Input: part model. Units: mm. Frame: model coordinates. A direction names the side the tool comes from. Round coordinates to 2 decimals unless told otherwise and drop trailing zeros. Order: outer loops, then holes, each group sorted by start corner. A loop starts at its lowest first (then second) coordinate and runs counter-clockwise, first axis right, second up. Notation, with made-up numbers: (50.5, 25) -> (64.5, 25) arc R7 ccw to (64.5, 38) -> close; hole circle Ø8 at (16.25, 64). An arc over 180 degrees is marked (long way). Use a Markdown table: item, result.
from build123d import *

# Parameters (mm, degrees)
SKETCH2_R                   = 7.9375
SKETCH2_R_2                 = 3.7465
BOSS_EXTRUDE1_DEPTH         = 204.47
FILLET1_R                   = 3.81
CIRPATTERN1_COUNT           = 4
FILLET1_OF_CIRPATTERN1_R    = 3.81
SKETCH3_R                   = 8.636
CUT_EXTRUDE1_DEPTH          = 12.7
CIRPATTERN2_COUNT           = 4
FILLET2_R                   = 2.54
MIRROR1_COPY_1_SKETCH_R     = 8.636
MIRROR1_COPY_1_DEPTH        = 12.7
MIRROR1_COPY_2_SKETCH_R     = 8.636
MIRROR1_COPY_2_DEPTH        = 12.7
MIRROR1_COPY_3_SKETCH_R     = 8.636
MIRROR1_COPY_3_DEPTH        = 12.7
FILLET3_R                   = 2.54
CHAMFER1_SIZE               = 1.27
CHAMFER1_SIZE_2             = 7.202527911
F_3_8_CLEARANCE_HOLE1_D     = 10.0838
F_3_8_CLEARANCE_HOLE1_DEPTH = 54.864
F_3_8_CLEARANCE_HOLE1_TIP   = 3.029479155
CIRPATTERN3_COUNT           = 3
CIRPATTERN3_ANGLE           = 180
CUT_EXTRUDE2_START          = -204.47
SKETCH9_R                   = 52.832
CUT_EXTRUDE2_DEPTH          = 101.788087
SKETCH10_W                  = 4.445
SKETCH10_H                  = 6.796913


with BuildPart() as part:
    # Sketch1 → Revolve1 (revolve)
    with BuildSketch(Plane.XY, mode=Mode.PRIVATE) as revolve1_sk:
        Polygon((44.45, 0), (44.45, 204.47), (50.7238, 204.47), (50.7238, 108.585), (52.832, 108.585), (52.832, 95.885), (50.7238, 95.885), (50.7238, 0), align=None)
    revolve(revolve1_sk.sketch.rotate(Axis((0, 138.931800571, 0), (0, -1, 0)), 180), axis=Axis((0, 138.931800571, 0), (0, -1, 0)))

    # Sketch2 → Boss-Extrude1 (add)
    with BuildSketch(Plane(origin=(0, 204.47, 0), x_dir=(1, 0, 0), z_dir=(0, 1, 0))):
        with Locations((0, 40.7035)):
            Circle(SKETCH2_R)
        with Locations(Location((0, 40.7035, 0), (0, 0, 180))):
            Circle(SKETCH2_R_2, mode=Mode.SUBTRACT)
    boss_extrude1 = extrude(amount=-BOSS_EXTRUDE1_DEPTH)

    # Fillet1
    fillet1_edges = [part.edges().sort_by_distance(p)[0] for p in [
        (-7.287865551, 102.235, -43.848483619),
        (7.287865551, 102.235, -43.848483619),
    ]]
    fillet(fillet1_edges, radius=FILLET1_R)

    # CirPattern1: Boss-Extrude1 ×4 about axis
    cirpattern1_axis = Axis((0, 0, 0), (0, 1, 0))
    for i in range(1, CIRPATTERN1_COUNT):
        add(boss_extrude1.rotate(cirpattern1_axis, i * 360 / CIRPATTERN1_COUNT))

    # Fillet1 of CirPattern1
    fillet1_of_cirpattern1_edges = [part.edges().sort_by_distance(p)[0] for p in [
        (-43.848483619, 102.235, 7.287865551),
        (-43.848483619, 102.235, -7.287865551),
        (7.287865551, 102.235, 43.848483619),
        (-7.287865551, 102.235, 43.848483619),
        (43.848483619, 102.235, -7.287865551),
        (43.848483619, 102.235, 7.287865551),
    ]]
    fillet(fillet1_of_cirpattern1_edges, radius=FILLET1_OF_CIRPATTERN1_R)

    # Sketch3 → Cut-Extrude1 (cut)
    with BuildSketch(Plane(origin=(0, 204.47, 0), x_dir=(1, 0, 0), z_dir=(0, 1, 0))):
        with Locations((0, 40.7035)):
            Circle(SKETCH3_R)
    cut_extrude1 = extrude(amount=-CUT_EXTRUDE1_DEPTH, mode=Mode.SUBTRACT)

    # CirPattern2: Cut-Extrude1 ×4 about axis
    cirpattern2_axis = Axis((0, 0, 0), (0, 1, 0))
    for i in range(1, CIRPATTERN2_COUNT):
        add(cut_extrude1.rotate(cirpattern2_axis, i * 360 / CIRPATTERN2_COUNT), mode=Mode.SUBTRACT)

    # Fillet2
    fillet2_edges = [part.edges().sort_by_distance(p)[0] for p in [
        (-8.61576795, 198.12, -41.294294914),
        (8.61576795, 198.12, -41.294294914),
        (-41.294294914, 198.12, 8.61576795),
        (8.61576795, 198.12, 41.294294914),
        (41.294294914, 198.12, -8.61576795),
        (41.294294914, 198.12, 8.61576795),
        (-8.61576795, 198.12, 41.294294914),
        (-41.294294914, 198.12, -8.61576795),
    ]]
    fillet(fillet2_edges, radius=FILLET2_R)

    # Mirror1: Cut-Extrude1 across plane
    add(cut_extrude1.mirror(Plane.ZX.offset(102.235)), mode=Mode.SUBTRACT)

    # Mirror1 copy 1 sketch → Mirror1 copy 1 (cut)
    with BuildSketch(Plane(origin=(0, 0, 0), x_dir=(0, 0, -1), z_dir=(0, -1, 0))):
        with Locations((0, -40.7035)):
            Circle(MIRROR1_COPY_1_SKETCH_R)
    extrude(amount=-MIRROR1_COPY_1_DEPTH, mode=Mode.SUBTRACT)

    # Mirror1 copy 2 sketch → Mirror1 copy 2 (cut)
    with BuildSketch(Plane(origin=(0, 0, 0), x_dir=(-1, 0, 0), z_dir=(0, -1, 0))):
        with Locations((0, -40.7035)):
            Circle(MIRROR1_COPY_2_SKETCH_R)
    extrude(amount=-MIRROR1_COPY_2_DEPTH, mode=Mode.SUBTRACT)

    # Mirror1 copy 3 sketch → Mirror1 copy 3 (cut)
    with BuildSketch(Plane(origin=(0, 0, 0), x_dir=(0, 0, 1), z_dir=(0, -1, 0))):
        with Locations((0, -40.7035)):
            Circle(MIRROR1_COPY_3_SKETCH_R)
    extrude(amount=-MIRROR1_COPY_3_DEPTH, mode=Mode.SUBTRACT)

    # Fillet3
    fillet3_edges = [part.edges().sort_by_distance(p)[0] for p in [
        (-41.294294914, 6.35, 8.61576795),
        (8.61576795, 6.35, 41.294294914),
        (41.294294914, 6.35, -8.61576795),
        (-8.61576795, 6.35, -41.294294914),
        (8.61576795, 6.35, -41.294294914),
        (41.294294914, 6.35, 8.61576795),
        (-8.61576795, 6.35, 41.294294914),
        (-41.294294914, 6.35, -8.61576795),
    ]]
    fillet(fillet3_edges, radius=FILLET3_R)

    # Chamfer1
    # the kernel refuses this chamfer: 7.202527911, 1.27 mm, written as the material it adds along each edge
    with BuildSketch(Plane(origin=(0, 95.885, 0), x_dir=(-1, 0, 0), z_dir=(0, 0, 1))) as chamfer1_piece_1_section:
        Polygon((50.7238, CHAMFER1_SIZE), (50.7238 + CHAMFER1_SIZE_2, 0), (50.7238, 0), align=None)
    chamfer1_piece_1 = revolve(axis=Axis((0, 95.885, 0), (0, -1, 0)), mode=Mode.PRIVATE)
    chamfer1_piece_1 = chamfer1_piece_1 & Plane(origin=(0, 94.871613174, 0), x_dir=(-1, 0, 0), z_dir=(0, -1, 0)) * Cylinder(52.832, 232, mode=Mode.PRIVATE)
    add(chamfer1_piece_1)

    # 3/8 Clearance Hole1
    with Locations(Plane(origin=(37.357865464, 0, 37.357865464), x_dir=(0, 1, 0), z_dir=(0.7071067811865488, 0, 0.7071067811865464))):
        with Locations((101.78586627, -9.525), (101.78586627, 9.525)):
            Hole(F_3_8_CLEARANCE_HOLE1_D / 2, depth=F_3_8_CLEARANCE_HOLE1_DEPTH)
            with Locations((0, 0, -(F_3_8_CLEARANCE_HOLE1_DEPTH + F_3_8_CLEARANCE_HOLE1_TIP / 2))):  # 118° drill point
                Cone(0, F_3_8_CLEARANCE_HOLE1_D / 2, F_3_8_CLEARANCE_HOLE1_TIP, mode=Mode.SUBTRACT)

    # Sketch8 → #6 Clearance Hole1 (revolve, cut)
    with BuildSketch(Plane(origin=(37.357865464, 101.78586627, -37.357865464), x_dir=(-0.7071067811865512, 0, -0.7071067811865438), z_dir=(0, 1, 0))):
        Polygon((0, 0), (0, 56.004824014), (1.89865, 54.864), (1.89865, 0), align=None)
    f_6_clearance_hole1 = revolve(axis=Axis((41.847993524, 101.78586627, -41.847993524), (-0.7071067811865438, 0, 0.7071067811865512)), mode=Mode.SUBTRACT)

    # CirPattern3: #6 Clearance Hole1 ×3 about axis
    cirpattern3_axis = Axis((0, 138.931800571, 0), (0, 1, 0))
    for i in range(1, CIRPATTERN3_COUNT):
        add(f_6_clearance_hole1.rotate(cirpattern3_axis, i * CIRPATTERN3_ANGLE / (CIRPATTERN3_COUNT - 1)), mode=Mode.SUBTRACT)

    # Sketch9 → Cut-Extrude2 (cut)
    with BuildSketch(Plane(origin=(0, 204.47, 0), x_dir=(1, 0, 0), z_dir=(0, 1, 0)).offset(CUT_EXTRUDE2_START)):
        with Locations(Location((0, 0, 0), (0, 0, 180))):
            Circle(SKETCH9_R)
    extrude(amount=CUT_EXTRUDE2_DEPTH, mode=Mode.SUBTRACT)

    # Sketch10 → Cut-Revolve1 (revolve, cut)
    with BuildSketch(Plane.XY, mode=Mode.PRIVATE) as cut_revolve1_sk:
        with Locations((50.6095, 105.1865435)):
            Rectangle(SKETCH10_W, SKETCH10_H)
    revolve(cut_revolve1_sk.sketch.rotate(Axis((0, 204.47, 0), (0, -1, 0)), 90), axis=Axis((0, 204.47, 0), (0, -1, 0)), mode=Mode.SUBTRACT)


solid = part.part
1) Draft query along Z for faces 4 (the face through (42, 101.788, -5)), 5 (the face through (0, 191.77, 45)), 6 (the face through (-47.975, 105.234, -6.299)). Return one class per face: released by +Z, released by -Z, zero draft, split by the parting line, or undercut.
Answer key:
| item | result |
|---|---|
| face 4 | zero draft |
| face 5 | undercut |
| face 6 | split by the parting line |
2) Ray query, probe 1 along Z at (x, y) = (3, 138) (3 decimals); probe 2 along X at (y, z) = (125, 36.5); probe 3 along X at (y, z) = (129, -25). Return the intervals inside material, ascending.
Answer key:
| item | result |
|---|---|
| probe 1 | z = -50.635 to -42.948, -38.459 to -33.355, 33.355 to 38.459, 42.948 to 50.635 |
| probe 2 | x = -35.22 to -25.37, -6.73 to 6.73, 25.37 to 35.22 |
| probe 3 | x = -44.14 to -36.75, 36.75 to 44.14 |
3) Cut plane A-A on x = 0. State how many separate pieces and enclosed holes the cut face has, and give its area (3 significant figures).
Answer key:
| item | result |
|---|---|
| separate pieces | 4 |
| enclosed holes | 0 |
| area | 1,890 mm^2 |
4) Set-up query: faces 1 (the face through (0.158, 147.409, 32.768)), 2 (the face through (-49.34, 198.21, -0.14)), 3 (the face through (-46, 101.788, 0)). Return all of +Z, -Z, +X, -X, +Y, -Y with unobstructed straight access to the full face (end or side cutting, diameter ignored); none if empty.
Answer key:
| item | result |
|---|---|
| face 1 | +Y, -Y |
| face 2 | +Y |
| face 3 | +Z, -Z, +X, -X, -Y |
5) Cut plane C-C on z = -21.5. Return loops of the section in (x, y) (3 decimals), and give its area (3 significant figures).
Answer key:
| item | result |
|---|---|
| outline | (-45.942, 108.585) -> (-43.348, 108.585) -> (-43.348, 101.788) -> (-38.904, 101.788) -> (-38.904, 204.47) -> (-45.942, 204.47) -> close; (38.904, 101.788) -> (43.348, 101.788) -> (43.348, 108.585) -> (45.942, 108.585) -> (45.942, 204.47) -> (38.904, 204.47) -> close |
| area | 1,410 mm^2 |
6) Contact query for flat-ended pins moving along their axis: P1, Ø2, axis at x = 31, y = 134, coming from the +Z side; P2, Ø6, axis at x = -1, y = 173, coming from the -Z side; P3, Ø5, axis at x = -39.5, z = -3, coming from the +Y side. Output: stop coordinate, or through.
Answer key:
| item | result |
|---|---|
| P1 | stops at z = 40.9 |
| P2 | stops at z = -50.72 |
| P3 | stops at y = 191.77 |
